Check sheet for the drawn part. Datum: minimum x, y, z corner. Units: mm. A direction names the side the tool comes from. Give positions to 0.01 mm unless a question says otherwise; leave off trailing zeros. Loops run counter-clockwise (first coordinate to the right, second up) from the corner with the lowest first, then second, coordinate; pieces in that order, holes last.
1. Go/stop test with flat-tipped pins: pin 1 Ø20 at (x, z) = (17.5, 21.67) entering from +Y; pin 2 Ø4 at (y, z) = (45.5, 21) entering from -X; pin 3 Ø18.5 at (y, z) = (21.25, 21.25) entering from +X; pin 4 Ø12 at (x, z) = (39.5, 16) entering from -Y. Record where each tip stops, or that it passes through.
2. Tool access check on the marked faces 4, 5, 6, 7 and 8. Record the directions out of +Z, -Z, +X, -X, +Y, -Y that give a thin tool (end or side, any length) a straight path to the whole face; none if there is none.
3. Cross-section at B-B, the plane x = 17.5. Record the cut outline in (y, z), plus the area to 3 significant figures.
4. Cross-section at A-A, the plane y = 21.25. Record the cut outline in (x, z).
5. Cross-section at D-D, the plane y = 7. Record the cut outline in (x, z).
6. Cross-section at C-C, the plane z = 23. Record the cut outline in (x, y), plus the area to 3 significant figures.
7. Material ranges on L1, parallel to Y at x = 68, z = 21; L2, parallel to X at y = 14.5, z = 32; L3, parallel to Z at x = 17, y = 77, recorded low to high.
8. Release check for a two-part mould opening along Z. For the marked faces 1, 2 and 3 record: +Z half, -Z half, draft (parallel to the pull), parting line (faces both ways), or undercut.
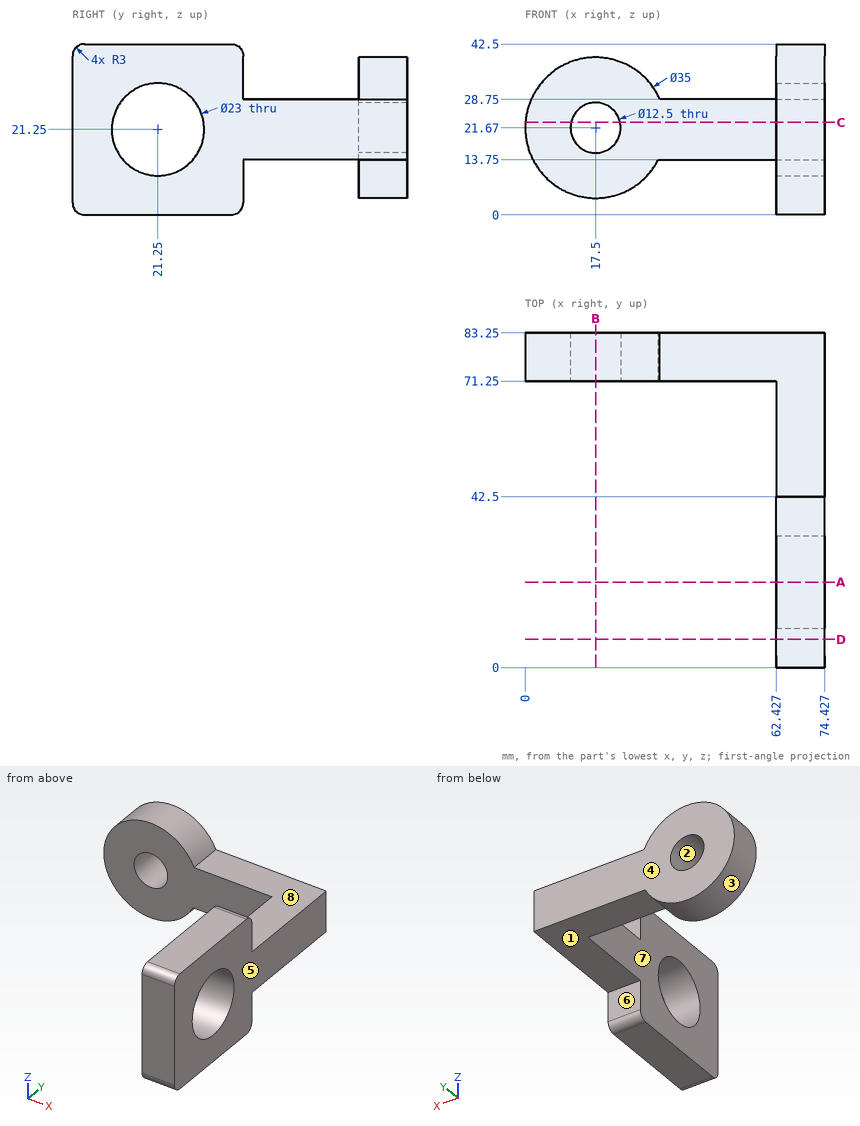
Result:
1. pin 1: stops at y = 83.25
1. pin 2: stops at x = 62.43
1. pin 3: passes through
1. pin 4: stops at y = 71.25
2. face 4: +Z, -Z, +X, -X, +Y
2. face 5: +Z, -Z, +X, +Y, -Y
2. face 6: -Z, +X, -X, +Y
2. face 7: +Z, -Z, -X, -Y
2. face 8: +Z, +X, +Y
3. outline: (71.25, 4.17) - (83.25, 4.17) - (83.25, 15.42) - (71.25, 15.42) - close; (71.25, 27.92) - (83.25, 27.92) - (83.25, 39.17) - (71.25, 39.17) - close
3. area: 270 mm2
4. outline: (62.43, 0) - (74.43, 0) - (74.43, 9.75) - (62.43, 9.75) - close; (62.43, 32.75) - (74.43, 32.75) - (74.43, 42.5) - (62.43, 42.5) - close
5. outline: (62.43, 0) - (74.43, 0) - (74.43, 42.5) - (62.43, 42.5) - close
6. outline: (0.05, 71.25) - (11.39, 71.25) - (11.39, 83.25) - (0.05, 83.25) - close; (23.61, 71.25) - (62.43, 71.25) - (62.43, 32.62) - (74.43, 32.62) - (74.43, 83.25) - (23.61, 83.25) - close; (62.43, 0) - (74.43, 0) - (74.43, 9.88) - (62.43, 9.88) - close
6. area: 1,330 mm2
7. L1: y = 0 to 9.75, 32.75 to 83.25
7. L2: x = 62.43 to 74.43
7. L3: z = 4.18 to 15.44, 27.9 to 39.16
8. face 1: -Z half
8. face 2: undercut
8. face 3: parting line
